Autodesk Inventor part; units mm, degrees
ref_plane "YZ Plane" through (0, 0, 0) normal (1, 0, 0) x (0, 1, 0)
ref_plane "XZ Plane" through (0, 0, 0) normal (0, 1, 0) x (-1, 0, 0)
ref_plane "XY Plane" through (0, 0, 0) normal (0, 0, 1) x (1, 0, 0)
sketch "Sketch1" plane through (0, 0, 0) normal (0, 0, 1) x (1, 0, 0)
  line L0 (-9, 10) -> (9, 10)
  line L1 (10, 9) -> (10, -9)
  line L2 (9, -10) -> (-9, -10)
  line L3 (-10, -9) -> (-10, 9)
  line L4 (-10, 10) -> (10, -10) construction
  line L5 (10, 10) -> (-10, -10) construction
  circle A0 centre (0, 0) radius 2
  line L6 (-4, 4) -> (4, 4)
  line L7 (4, 4) -> (4, -4)
  line L8 (4, -4) -> (-4, -4)
  line L9 (-4, -4) -> (-4, 4)
  line L10 (-4, 4) -> (4, -4) construction
  line L11 (4, 4) -> (-4, -4) construction
  arc A1 (-9, 10) -> (-10, 9) centre (-9, 9) ccw
  arc A2 (10, 9) -> (9, 10) centre (9, 9) ccw
  arc A3 (9, -10) -> (10, -9) centre (9, -9) ccw
  arc A4 (-10, -9) -> (-9, -10) centre (-9, -9) ccw
  line L12 (-3.1, 10) -> (3.1, 10)
  line L13 (3.1, 10) -> (3.1, -10)
  line L14 (3.1, -10) -> (-3.1, -10)
  line L15 (-3.1, -10) -> (-3.1, 10)
  line L16 (-10, 3.1) -> (10, 3.1)
  line L17 (10, 3.1) -> (10, -3.1)
  line L18 (10, -3.1) -> (-10, -3.1)
  line L19 (-10, -3.1) -> (-10, 3.1)
  line L20 (-5.5, 10) -> (5.5, 10)
  line L21 (5.5, 10) -> (5.5, -10)
  line L22 (5.5, -10) -> (-5.5, -10)
  line L23 (-5.5, -10) -> (-5.5, 10)
  line L24 (-10, 5.5) -> (10, 5.5)
  line L25 (10, 5.5) -> (10, -5.5)
  line L26 (10, -5.5) -> (-10, -5.5)
  line L27 (-10, -5.5) -> (-10, 5.5)
  line L28 (-8.3, 5.5) -> (-8.3, 3.1)
  line L29 (-8.3, -5.5) -> (-8.3, -3.1)
  line L30 (8.3, -5.5) -> (8.3, -3.1)
  line L31 (8.3, 5.5) -> (8.3, 3.1)
  line L32 (-5.5, 8.3) -> (-3.1, 8.3)
  line L33 (3.1, 8.3) -> (5.5, 8.3)
  line L34 (-5.5, -8.3) -> (-3.1, -8.3)
  line L35 (3.1, -8.3) -> (5.5, -8.3)
  line L36 (-4, 2.5) -> (-7, 5.5)
  line L37 (-4, 2.5) -> (0.2426, 2.5) construction
  line L38 (-4, -2.5) -> (-7, -5.5)
  line L39 (-4, -2.5) -> (0.2426, -2.5) construction
  line L40 (-2.5, 4) -> (-5.5, 7)
  line L41 (-2.5, 4) -> (1.7426, 4) construction
  line L42 (5.5, 7) -> (2.5, 4)
  line L43 (5.5, 7) -> (9.7426, 7) construction
  line L44 (7, 5.5) -> (4, 2.5)
  line L45 (7, 5.5) -> (11.2426, 5.5) construction
  line L46 (7, -5.5) -> (4, -2.5)
  line L47 (7, -5.5) -> (11.2426, -5.5) construction
  line L48 (2.5, -4) -> (5.5, -7)
  line L49 (2.5, -4) -> (6.7426, -4) construction
  line L50 (-2.5, -4) -> (-5.5, -7)
  line L51 (-2.5, -4) -> (1.7426, -4) construction
  point P0 (3.1, -3.1)
  point P1 (3.1, -5.5)
  point P2 (5.5, -5.5)
  point P3 (10, 3.1)
  point P4 (-5.5, -5.5)
  point P5 (-3.1, -5.5)
  point P6 (-3.1, -3.1)
  dimension "d0" = 20
  dimension "d1" = 20
  dimension "d2" = 4
  dimension "d3" = 8
  dimension "d4" = 8
  dimension "d5" = 1
  dimension "d6" = 6.2
  dimension "d7" = 3.1
  dimension "d8" = 6.2
  dimension "d9" = 3.1
  dimension "d10" = 11
  dimension "d11" = 5.5
  dimension "d12" = 11
  dimension "d13" = 5.5
  dimension "d14" = 4.3
  dimension "d15" = 4.3
  dimension "d16" = 4.3
  dimension "d17" = 4.3
  dimension "d18" = 135
  dimension "d19" = 135
  dimension "d20" = 135
  dimension "d21" = 135
  dimension "d22" = 135
  dimension "d23" = 135
  dimension "d24" = 1.3
  dimension "d25" = 1.3
  dimension "d26" = 1.3
  dimension "d27" = 1.3
  dimension "d28" = 1.3
  dimension "d29" = 1.3
  dimension "d32" = 45
  dimension "d33" = 135
  dimension "d34" = 1.3
  dimension "d35" = 1.3
extrude "Extrusion1" add sketch "Sketch1" along normal blind 20 contours L0 L23 L24 L3 A1 | L0 L15 L32 L23 | L24 L28 L16 L3 | L0 L21 L33 L13 | L40 L24 L23 | L0 A2 L1 L24 L21 | L24 L40 L15 L6 L9 L16 L36 L23 | L23 L36 L24 | L18 L29 L26 L3 | L40 L6 L15 | L26 L23 L2 A4 L3 | L21 L24 L42 | L42 L24 L21 L44 L16 L7 L6 L13 | L13 L6 L42 | L15 L16 L9 L6 | L6 L13 L16 L15 | L16 L9 L36 | L1 L16 L31 L24 | L24 L44 L21 | L6 L7 L16 L13 | L16 L13 L18 L15 | L15 L18 L9 L16 | L38 L23 L26 | L38 L9 L18 | L18 L9 L8 L15 L50 L26 L23 L38 | L16 L7 L18 L13 | L18 L13 L8 L15 | L15 L8 L9 L18 | L23 L34 L15 L2 | L26 L50 L23 | L1 L26 L30 L18 | L44 L7 L16 | L18 L7 L8 L13 | L8 L50 L15 | L1 A3 L2 L21 L26 | L13 L48 L8 | L8 L7 L18 L46 L21 L26 L48 L13 | L7 L46 L18 | L13 L35 L21 L2 | L46 L26 L21 | L21 L48 L26
equation "\"d7\" = 0.5 * d6"
equation "\"d8\" = d6"
equation "\"d11\" = 0.5 * d10"
equation "\"d12\" = d10"
properties part number "Aluminum_Profile_202020"
For this review, take the finished solid that the model builds, in its own axes (mm). A direction names the side the tool comes from. Round coordinates to 2 decimals unless told otherwise and drop trailing zeros. Order: outer loops, then holes, each group sorted by start corner. A loop starts at its lowest first (then second) coordinate and runs counter-clockwise, first axis right, second up. Notation, with made-up numbers: (75, 62.25) -> (96, 62.25) arc R14 ccw to (96, 72.25) -> close; hole circle Ø11 at (82.5, 63). An arc over 180 degrees is marked (long way). Write item = value, one per line. Start each with the question number.
1) Take a section at C-C on x = 3.5. State the section outline as (y, z) points.
2) Tool access review of faces 5 (the face through (-9, -3.1, 10)), 6 (the face through (4, 5.5, 9.9)), 7 (the face through (4, 0, 10)): name each direction out of +Z, -Z, +X, -X, +Y, -Y from which nothing blocks a thin tool from reaching the whole face with its end or side.
3) Insertion check: pin 1 (0.8 mm diameter, centred on x = 9.5, z = 14.5, fed in from -Y) (3 decimals); pin 2 (2.5 mm diameter, centred on x = 0, z = 14.5, fed in from -Y); pin 3 (2.5 mm diameter, centred on y = 0, z = 11, fed in from -X). Each pin has a flat end and moves straight along its axis. Give the tip position at first contact, or say it passes through.
4) Take a section at D-D on y = 5. State the section outline as (x, z) points, plus the area to 3 significant figures.
5) Take a section at B-B on x = 0. State the section outline as (y, z) points, plus the area to 3 significant figures.
6) To check wall thickness, follow line 1 (X direction, y = -8, z = 7); line 2 (Y direction, x = 0, z = 4); line 3 (X direction, y = 4.75, z = 11.5). State the ranges of each line that lie inside material, in increasing order. Write a range as from..to.
7) The part is to be moulded in two halves that separate along Y. For faces 1 (the face through (-9.715, 9.699, 9.86)), 2 (the face through (4, -8.3, 10)), 3 (the face through (3.1, -9, 10)), 4 (the face through (5.5, 8, 10)), say which applies: +Y half, -Y half, draft (parallel to the pull), parting line (faces both ways), or undercut.
8) Take a section at A-A on y = -6.25. State the section outline as (x, z) points.
Verdict:
q1.outline = (-10, 0) -> (-8.3, 0) -> (-8.3, 20) -> (-10, 20) -> close; (-5, 0) -> (5, 0) -> (5, 20) -> (-5, 20) -> close; (8.3, 0) -> (10, 0) -> (10, 20) -> (8.3, 20) -> close
q2.face_5 = +Z, -Z, -X
q2.face_6 = +Z, -Z
q2.face_7 = +Z, -Z, +X
q3.pin_1 = -9.995
q3.pin_2 = -4
q3.pin_3 = -4
q4.outline = (-10, 0) -> (-8.3, 0) -> (-8.3, 20) -> (-10, 20) -> close; (-6.5, 0) -> (-3.5, 0) -> (-3.5, 20) -> (-6.5, 20) -> close; (3.5, 0) -> (6.5, 0) -> (6.5, 20) -> (3.5, 20) -> close; (8.3, 0) -> (10, 0) -> (10, 20) -> (8.3, 20) -> close
q4.area = 188 mm2
q5.outline = (-4, 0) -> (-2, 0) -> (-2, 20) -> (-4, 20) -> close; (2, 0) -> (4, 0) -> (4, 20) -> (2, 20) -> close
q5.area = 80.0 mm2
q6.line_1 = -10..-5.5, 5.5..10
q6.line_2 = -4..-2, 2..4
q6.line_3 = -10..-8.3, -6.25..-3.25, 3.25..6.25, 8.3..10
q7.face_1 = +Y half
q7.face_2 = undercut
q7.face_3 = draft
q7.face_4 = undercut
q8.outline = (-10, 0) -> (-4.75, 0) -> (-4.75, 20) -> (-10, 20) -> close; (4.75, 0) -> (10, 0) -> (10, 20) -> (4.75, 20) -> close
